Model file for the job. Use its own axes, mm. Round coordinates to 2 decimals unless told otherwise and drop trailing zeros. Order: outer loops, then holes, each group sorted by start corner. A loop starts at its lowest first (then second) coordinate and runs counter-clockwise, first axis right, second up. Notation, with made-up numbers: (-36.75, -15.5) -> (-7.75, -15.5) arc R12 ccw to (-7.75, -8.5) -> close; hole circle Ø1 at (-30, 23). An arc over 180 degrees is marked (long way). Use CSV: the item, a comma, the result in double quotes.
```python
from build123d import *

# Parameters (mm, degrees)
F0_R     = 76.2
F2_DEPTH = 6.35
F1_R     = 3.175
F3_DEPTH = 6.35


with BuildPart() as f2:
    # F0 (on Top) → F2 (new body, symmetric)
    with BuildSketch(Plane.XY):
        Circle(F0_R)
    extrude(amount=F2_DEPTH, both=True)

    # F1 (on Top) → F3 (cut, symmetric)
    with BuildSketch(Plane.XY):
        with Locations((0, 63.5)):
            Circle(F1_R)
        with Locations((63.5, 0)):
            Circle(F1_R)
        with Locations((-63.5, 0)):
            Circle(F1_R)
        with Locations((0, -63.5)):
            Circle(F1_R)
        with Locations((-44.901281, 44.901281)):
            Circle(F1_R)
        with Locations((44.901281, 44.901281)):
            Circle(F1_R)
        with Locations((44.901281, -44.901281)):
            Circle(F1_R)
        with Locations((-44.901281, -44.901281)):
            Circle(F1_R)
    extrude(amount=F3_DEPTH, both=True, mode=Mode.SUBTRACT)


solid = f2.part
```
Q1. Cut at A-A (y = 0). Give the cut face in (x, z) (3 decimals).
From the geometry:
outline,"(-76.2, -6.35) -> (-66.675, -6.35) -> (-66.675, 6.35) -> (-76.2, 6.35) -> close; (-60.325, -6.35) -> (60.325, -6.35) -> (60.325, 6.35) -> (-60.325, 6.35) -> close; (66.675, -6.35) -> (76.2, -6.35) -> (76.2, 6.35) -> (66.675, 6.35) -> close"
Q2. Mould opens along Y. For faces 1 (the cylindrical face through (-60.47, -46.367, 0.089)), 2 (the flat face through (-1, 1, -6.35)), 3 (the cylindrical face through (-45.6, -48, 0.1)) say: +Y half, -Y half, draft (parallel to the pull), parting line (faces both ways), or undercut.
From the geometry:
face 1,"parting line"
face 2,"draft"
face 3,"undercut"
Q3. Pin check, flat tips, straight feed: pin 1 (5 mm diameter, centred on x = -22, z = -1, fed in from +Y); pin 2 (4 mm diameter, centred on x = 15.5, z = 0, fed in from +Y); pin 3 (4 mm diameter, centred on x = 21.5, z = -4, fed in from -Y). Stop position of each tip, or through.
From the geometry:
pin 1,"stops at y = 73.66"
pin 2,"stops at y = 74.99"
pin 3,"stops at y = -73.66"
Q4. Cut at B-B (y = -63.5). Give the cut face in (x, z) (3 decimals), plus the area to 3 significant figures.
From the geometry:
outline,"(-42.121, -6.35) -> (-3.175, -6.35) -> (-3.175, 6.35) -> (-42.121, 6.35) -> close; (3.175, -6.35) -> (42.121, -6.35) -> (42.121, 6.35) -> (3.175, 6.35) -> close"
area,"989 mm²"
Q5. Cut at D-D (x = -46). Give the cut face in (y, z).
From the geometry:
outline,"(-60.75, -6.35) -> (-47.88, -6.35) -> (-47.88, 6.35) -> (-60.75, 6.35) -> close; (-41.92, -6.35) -> (41.92, -6.35) -> (41.92, 6.35) -> (-41.92, 6.35) -> close; (47.88, -6.35) -> (60.75, -6.35) -> (60.75, 6.35) -> (47.88, 6.35) -> close"
Q6. Probe line 1 along Y through (x, z) = (0, -4) (3 decimals); line 2 along Y through (x, z) = (0.5, 2.5); line 3 along X through (y, z) = (64, -4). List the from-to ranges inside material, lowest first.
From the geometry:
line 1,"y = -76.2 to -66.675, -60.325 to 60.325, 66.675 to 76.2"
line 2,"y = -76.2 to -66.64, -60.36 to 60.36, 66.64 to 76.2"
line 3,"x = -41.36 to -3.14, 3.14 to 41.36"
